Build history of the part. All positions in model axes, mm. A direction names the side the tool comes from. Round coordinates to 2 decimals unless told otherwise and drop trailing zeros. Loops run counter-clockwise (first coordinate to the right, second up) from the corner with the lowest first, then second, coordinate; pieces in that order, holes last. Notation, with made-up numbers: (-29, 25.5) -> (3, 25.5) arc R18 ccw to (3, 30.5) -> close; hole circle Ø2 at (89.25, 76.25). An arc over 180 degrees is marked (long way). Put each result on its own line as item: value. Start each with the question number.
```python
from build123d import *

# Parameters (mm, degrees)
F0_R     = 18.034
F1_DEPTH = 30.9372
F2_T     = -2.54
F0_W     = 55.88
F0_H     = 55.88
F3_DEPTH = 12.7


with BuildPart() as f1:
    # F0 (on Top) → F1 (new body)
    with BuildSketch(Plane.XY):
        Circle(F0_R)
    extrude(amount=-F1_DEPTH)

    # F2
    f2_openings = [f1.faces().sort_by_distance(p)[0] for p in [
        (0, 0, 0),
    ]]
    offset(amount=F2_T, openings=f2_openings)

    # F0 (on Top) → F3 (join)
    with BuildSketch(Plane.XY):
        Rectangle(F0_W, F0_H)
        Circle(F0_R, mode=Mode.SUBTRACT)
        Circle(F0_R)
    extrude(amount=F3_DEPTH)


solid = f1.part
```
Item 1: Pull direction Y, two halves, no side cores. Call faces 1 (the face through (0, 0, -28.397)), 2 (the face through (-3.909, -17.605, -15.252)), 3 (the face through (0, 0, 12.7)): +Y half, -Y half, draft (parallel to the pull), parting line (faces both ways), or undercut.
Item 2: Drop flat-ended pins along their axis: pin 1 (4 mm diameter, centred on x = -3.5, z = -3.5, fed in from +Y); pin 2 (4 mm diameter, centred on x = -10.5, z = -13, fed in from +Y); pin 3 (8 mm diameter, centred on x = 19.5, z = -18, fed in from +Y). Give the stop position or say it passes through.
Item 3: 3-axis set-ups, long thin cutter, end or side, ignore diameter. For faces 4 (the face through (-13, 13, 0)), 5 (the face through (-27.94, 0, 6)), 6 (the face through (0, 0, 0)): which of +Z, -Z, +X, -X, +Y, -Y reach the whole face in a straight line?
Item 4: Cut at D-D on y = 17. Write the cut outline in (x, z), then the cut area to 3 significant figures.
Item 5: Wall check: line 1 (Y direction, x = 0, z = -15.5); line 2 (Z direction, x = -21.5, y = -19.5); line 3 (Z direction, x = 4, y = -12). Give the ranges that are in metal, low to high. Write a range as from..to.
Item 6: Cut at A-A on x = 0. Write the cut outline in (y, z).
Item 7: Cut at C-C on z = -20.5. Write the cut outline in (x, y).
Ans:
1. face 1: undercut
1. face 2: parting line
1. face 3: draft
2. pin 1: stops at y = 17.97
2. pin 2: stops at y = 15.91
2. pin 3: stops at y = 9.22
3. face 4: -Z
3. face 5: +Z, -Z, -X, +Y, -Y
3. face 6: none
4. outline: (-27.94, 0) -> (-6.02, 0) -> (-6.02, -30.94) -> (6.02, -30.94) -> (6.02, 0) -> (27.94, 0) -> (27.94, 12.7) -> (-27.94, 12.7) -> close
4. area: 1,080 mm2
5. line 1: y = -18.03..-15.49, 15.49..18.03
5. line 2: z = 0..12.7
5. line 3: z = -30.94..-28.4, 0..12.7
6. outline: (-27.94, 0) -> (-18.03, 0) -> (-18.03, -30.94) -> (18.03, -30.94) -> (18.03, 0) -> (27.94, 0) -> (27.94, 12.7) -> (-27.94, 12.7) -> close; hole (-15.49, -28.4) -> (15.49, -28.4) -> (15.49, 0) -> (-15.49, 0) -> close
7. outline: circle Ø36.07 at (0, 0); hole circle Ø30.99 at (0, 0)
